from build123d import *

# Parameters (mm, degrees)
SKETCH1_W           = 12.7
SKETCH1_H           = 19.05
BOSS_EXTRUDE1_DEPTH = 10.414
SKETCH2_W           = 10.7
SKETCH2_H           = 17.05
CUT_EXTRUDE1_DEPTH  = 2.414
SKETCH4_W           = 1.5
SKETCH4_H           = 16.05
CUT_EXTRUDE2_DEPTH  = 42.414
SKETCH5_W           = 1.5
SKETCH5_H           = 9.7
CUT_EXTRUDE3_DEPTH  = 42.414
CUT_EXTRUDE4_DEPTH  = 0.2


with BuildPart() as part:
    # Sketch1 → Boss-Extrude1 (new body)
    with BuildSketch(Plane.YZ):
        with Locations((10.524991597, -9.20910084)):
            Rectangle(SKETCH1_W, SKETCH1_H)
    extrude(amount=BOSS_EXTRUDE1_DEPTH)

    # Sketch2 → Cut-Extrude1 (cut)
    with BuildSketch(Plane(origin=(0, 0, 0), x_dir=(0, -1, 0), z_dir=(-1, 0, 0))):
        with Locations((-10.524991597, -9.20910084)):
            Rectangle(SKETCH2_W, SKETCH2_H)
    extrude(amount=-CUT_EXTRUDE1_DEPTH, mode=Mode.SUBTRACT)

    # Sketch4 → Cut-Extrude2 (cut)
    with BuildSketch(Plane(origin=(0, 16.874991597, 0), x_dir=(-1, 0, 0), z_dir=(0, 1, 0))):
        with Locations((-0.75, -9.20910084)):
            Rectangle(SKETCH4_W, SKETCH4_H)
    extrude(amount=-CUT_EXTRUDE2_DEPTH, mode=Mode.SUBTRACT)

    # Sketch5 → Cut-Extrude3 (cut)
    with BuildSketch(Plane(origin=(0, 0, -18.73410084), x_dir=(1, 0, 0), z_dir=(0, 0, -1))):
        with Locations((0.75, -10.524991597)):
            Rectangle(SKETCH5_W, SKETCH5_H)
    extrude(amount=-CUT_EXTRUDE3_DEPTH, mode=Mode.SUBTRACT)

    # Sketch6 → Cut-Extrude4 (cut)
    with BuildSketch(Plane.YZ.offset(10.414)):
        Polygon((7.471753677, -14.994134662), (13.347648049, -14.994134662), (14.427648049, -16.074134662), (6.391753677, -16.074134662), align=None)
        Polygon((14.427648049, -1.772534662), (6.391753677, -1.772534662), (7.471753677, -2.852534662), (13.347648049, -2.852534662), align=None)
        Polygon((13.432500863, -14.909281848), (13.432500863, -9.548187475), (13.972500863, -9.008187475), (14.512500863, -9.548187475), (14.512500863, -15.989281848), align=None)
        Polygon((7.386900863, -2.937387475), (6.306900863, -1.857387475), (6.306900863, -8.298481848), (6.846900863, -8.838481848), (7.386900863, -8.298481848), align=None)
        Polygon((13.432500863, -2.937387475), (14.512500863, -1.857387475), (14.512500863, -8.298481848), (13.972500863, -8.838481848), (13.432500863, -8.298481848), align=None)
        Polygon((7.471753677, -8.383334662), (13.347648049, -8.383334662), (13.887648049, -8.923334662), (13.347648049, -9.463334662), (7.471753677, -9.463334662), (6.931753677, -8.923334662), align=None)
        Polygon((6.846900863, -9.008187475), (6.306900863, -9.548187475), (6.306900863, -15.989281848), (7.386900863, -14.909281848), (7.386900863, -9.548187475), align=None)
    extrude(amount=-CUT_EXTRUDE4_DEPTH, mode=Mode.SUBTRACT)


solid = part.part
The listing builds one solid part. Answer for the finished solid, in the listing's coordinates (mm). A direction names the side the tool comes from. Coordinates: 2 decimals unless noted, no trailing zeros. Order: outer loops, then holes, each group sorted by start corner. A loop starts at its lowest first (then second) coordinate and runs counter-clockwise, first axis right, second up.
Q1. A cutting plane is placed at A-A, the plane x = 1. Write down the section's boundary in (y, z) (3 decimals).
Q2. Which of the six approach directions +Z, -Z, +X, -X, +Y, -Y give full straight-line access (tool end or side, diameter ignored) to faces 1 (the face through (1.5, 16.4, -9.3)), 2 (the face through (0, 16, -18)), 3 (the face through (10.214, 14, -5)), 4 (the face through (1, 5.675, -18)), 5 (the face through (2, 5.175, -9))?
Q3. A cutting plane is placed at D-D, the plane z = -16.75. Write down the section's boundary in (x, y) (3 decimals), and give its area (3 significant figures).
Q4. A cutting plane is placed at C-C, the plane y = 9.5. Write down the section's boundary in (x, z).
Q5. Given P1, Ø4, axis at y = 12, z = -3.5, coming from the -X side; P2, Ø0.9, axis at y = 9, z = -15.5, coming from the +X side, each flat-ended and moving along its own axis, determine where each tip first touches the part or whether it passes through.
Q6. Consider line 1 (Z direction, x = 2.25, y = 11.5); line 2 (Y direction, x = 1.75, z = -1) (3 decimals); line 3 (X direction, y = 7.5, z = -13.5). Determine where each line is inside the solid, lowest interval first.
Q7. For a pull along Y with two mould halves and no side action, classify faces 6 (the face through (0.8, 16.4, -1.184)), 7 (the face through (10.214, 7, -12)), 8 (the face through (5, 4.175, -9)) as pulls with the +Y half, pulls with the -Y half, needs draft (parallel to the pull), parting line crosses it, or undercut.
Answers follow:
1. outline: (4.175, -18.734) - (5.675, -18.734) - (5.675, -17.734) - (5.175, -17.734) - (5.175, -17.234) - (4.175, -17.234) - close; (4.175, -1.184) - (5.175, -1.184) - (5.175, -0.684) - (5.675, -0.684) - (5.675, 0.316) - (4.175, 0.316) - close; (15.375, -18.734) - (16.875, -18.734) - (16.875, -17.234) - (15.875, -17.234) - (15.875, -17.734) - (15.375, -17.734) - close; (15.375, -0.684) - (15.875, -0.684) - (15.875, -1.184) - (16.875, -1.184) - (16.875, 0.316) - (15.375, 0.316) - close
2. face 1: -X, +Y, -Y
2. face 2: +Z, -Z, -X, +Y, -Y
2. face 3: +X
2. face 4: +Z, -Z, -X
2. face 5: -X
3. outline: (1.5, 4.175) - (10.414, 4.175) - (10.414, 16.875) - (1.5, 16.875) - (1.5, 15.875) - (2.414, 15.875) - (2.414, 5.175) - (1.5, 5.175) - close
3. area: 103 mm2
4. outline: (1.5, -18.73) - (10.41, -18.73) - (10.41, -16.07) - (10.21, -16.07) - (10.21, -14.99) - (10.41, -14.99) - (10.41, -9.46) - (10.21, -9.46) - (10.21, -8.38) - (10.41, -8.38) - (10.41, -2.85) - (10.21, -2.85) - (10.21, -1.77) - (10.41, -1.77) - (10.41, 0.32) - (1.5, 0.32) - (1.5, -0.68) - (2.41, -0.68) - (2.41, -17.73) - (1.5, -17.73) - close
5. P1: stops at x = 2.41
5. P2: stops at x = 10.21
6. line 1: z = -18.73 to -17.73, -0.68 to 0.32
6. line 2: y = 4.175 to 5.175, 15.875 to 16.875
6. line 3: x = 2.41 to 10.41
7. face 6: needs draft
7. face 7: undercut
7. face 8: pulls with the -Y half
